Autodesk Inventor part; units mm, degrees
ref_plane "YZ Plane" through (0, 0, 0) normal (1, 0, 0) x (0, 1, 0)
ref_plane "XZ Plane" through (0, 0, 0) normal (0, 1, 0) x (-1, 0, 0)
ref_plane "XY Plane" through (0, 0, 0) normal (0, 0, 1) x (1, 0, 0)
sketch "Эскиз1" plane through (0, 0, 0) normal (0, 1, 0) x (-1, 0, 0)
  line L0 (0, 0) -> (4.25, 0)
  line L1 (4.25, 0) -> (4.25, -2)
  line L2 (0, -2) -> (2.5, -2)
  line L3 (2.5, -2.6792) -> (2.5, -10)
  line L4 (2.5, -10) -> (0, -10)
  line L5 (0, -10) -> (0, -2)
  line L6 (2.5, -2) -> (3, -2)
  line L7 (3, -2) -> (3, -2.6792)
  line L8 (3, -2.6792) -> (2.5, -2.6792)
  line L9 (3, -2) -> (4.25, -2)
  line L10 (0, 0) -> (0, -2)
  dimension "d0" = 4.25
  dimension "d1" = 2
  dimension "d3" = 8
  dimension "d4" = 0.5
revolve "Вращение1" add sketch "Эскиз1" angle 360 about axis through (0, 0, -10) along (0, 0, 1)
thread "Резьба1"
chamfer "Фаска1" distance 0.5 angle 45 1 edges at (2.5, 0, -10)
properties part number "Болт штурвал"
Geometry check sheet. Reference: the model listing, model coordinates, mm. A direction names the side the tool comes from. Round coordinates to 2 decimals unless told otherwise and drop trailing zeros. Order: outer loops, then holes, each group sorted by start corner. A loop starts at its lowest first (then second) coordinate and runs counter-clockwise, first axis right, second up. Notation, with made-up numbers: (37.25, 33.25) -> (42.25, 33.25) arc R17 cw to (42.25, 54.25) -> close; hole circle Ø8 at (-3.75, 12.25). An arc over 180 degrees is marked (long way). Use one line per item in the form item = value.
1. Cross-section at D-D, the plane z = -5.5. Enter the section's corners in (x, y), plus the area to 3 significant figures.
Working result:
outline = circle Ø5 at (0, 0)
area = 19.6 mm^2
2. Cross-section at C-C, the plane z = -2.5. Enter the section's corners in (x, y), plus the area to 3 significant figures.
Working result:
outline = circle Ø6 at (0, 0)
area = 28.3 mm^2
3. Cross-section at A-A, the plane x = 0. Enter the section's corners in (y, z), plus the area to 3 significant figures.
Working result:
outline = (-4.25, -2) -> (-3, -2) -> (-3, -2.68) -> (-2.5, -2.68) -> (-2.5, -9.5) -> (-2, -10) -> (2, -10) -> (2.5, -9.5) -> (2.5, -2.68) -> (3, -2.68) -> (3, -2) -> (4.25, -2) -> (4.25, 0) -> (-4.25, 0) -> close
area = 57.4 mm^2
4. Set-up check for faces 1 (the face through (2, -2, -2.679)), 2 (the face through (-2.285, 3.584, -1.014)): record each of +Z, -Z, +X, -X, +Y, -Y from which the full face is reachable in a straight line by a thin tool's end or side.
Working result:
face_1 = -Z
face_2 = +Z, -Z
5. Go/stop test with flat-tipped pins: pin 1 (3 mm diameter, centred on x = -2, z = -1.5, fed in from +Y); pin 2 (4 mm diameter, centred on y = 0, z = -8, fed in from +X); pin 3 (2 mm diameter, centred on y = -2, z = -2, fed in from -X). Record where each tip stops, or that it passes through.
Working result:
pin_1 = 4.22
pin_2 = 2.5
pin_3 = -4.13
6. Scan lines: line 1 along X through (y, z) = (1.5, -4.5); line 2 along Z through (x, y) = (-3.5, -2); line 3 along Z through (x, y) = (-1.75, -2.25). Record each from-to range of solid material in increasing order. Write a range as from..to.
Working result:
line_1 = -2..2
line_2 = -2..0
line_3 = -2.68..0
